Check sheet for the modelled part. Datum: model origin and axes. Units: mm. Face numbers are marked on the shaded views. A direction names the side the tool comes from. Give positions to 0.01 mm unless a question says otherwise; leave off trailing zeros. Loops run counter-clockwise (first coordinate to the right, second up) from the corner with the lowest first, then second, coordinate; pieces in that order, holes last. Notation, with made-up numbers: (-1.5, 11) -> (12.5, 11) arc R30 cw to (12.5, 47) -> close; hole circle Ø7 at (-5.75, 59.5). An arc over 180 degrees is marked (long way). Write each question's results on one line, items separated by ' | '. Start each with the question number.
Item 1: Scan lines: line 1 along Y through (x, z) = (23.5, 33); line 2 along Y through (x, z) = (1, 16); line 3 along Z through (x, y) = (-7, -13). Record each from-to range of solid material in increasing order.
Item 2: Cross-section at B-B on z = -7.5. Enter the section's corners in (x, y).
Item 3: Cross-section at C-C on x = 12.5. Enter the section's corners in (y, z).
Item 4: Access from +Z, -Z, +X, -X, +Y, -Y to the whole of each face (thin tool, end or side, straight path). Record for the marked faces 5, 6 and 7.
Item 5: Gauge pin test, flat ends, axial feed: pin 1 Ø6 at (y, z) = (-11.14, -7.5) entering from +X; pin 2 Ø0.9 at (x, y) = (33.5, -23) entering from +Z; pin 3 Ø7.5 at (x, z) = (30.5, -9) entering from +Y; pin 4 Ø3 at (x, z) = (33.81, -7.5) entering from -Y. Record the tip position at first contact, or that the pin passes through.
Item 6: Cross-section at D-D on z = 5.5. Enter the section's corners in (x, y), then the cut area to 3 significant figures.
Item 7: Cross-section at A-A on z = 39.5. Enter the section's corners in (x, y).
Item 8: Mould release check, pull along Y, two halves, no side actions. Record for the marked faces 1, 2, 3 and 4: pulls with the +Y half, pulls with the -Y half, needs draft (parallel to the pull), parting line crosses it, or undercut.
from build123d import *

# Parameters (mm, degrees)
SKETCH_1_W          = 42
SKETCH_1_H          = 61.5
EXTRUDE_1_DEPTH     = 3
SKETCH_2_W          = 42
SKETCH_2_H          = 9.2
SKETCH_2_H_2        = 2
EXTRUDE_2_DEPTH     = 42
SKETCH_3_R          = 12
SKETCH_3_R_2        = 1.65
CUT_EXTRUDE_1_DEPTH = 3
EXTRUDE_3_DEPTH     = 15
SKETCH_6_R          = 2.65
CUT_EXTRUDE_2_DEPTH = 5
SKETCH_7_W          = 15
SKETCH_7_H          = 3
EXTRUDE_4_DEPTH     = 20
SKETCH_8_R          = 2.65
CUT_EXTRUDE_3_DEPTH = 20


with BuildPart() as part:
    # 草图1 → 凸台-拉伸1 (new body)
    with BuildSketch(Plane.XY):
        with Locations((2.806034483, -19.390086207)):
            Rectangle(SKETCH_1_W, SKETCH_1_H)
    extrude(amount=EXTRUDE_1_DEPTH)

    # 草图2 → 凸台-拉伸2 (add)
    with BuildSketch(Plane.XY.offset(3)):
        with Locations((2.806034483, -45.540086207)):
            Rectangle(SKETCH_2_W, SKETCH_2_H)
        with Locations((2.806034483, 10.359913793)):
            Rectangle(SKETCH_2_W, SKETCH_2_H_2)
    extrude(amount=EXTRUDE_2_DEPTH)

    # 草图3 → 切除-拉伸1 (cut, through all)
    with BuildSketch(Plane.XZ.offset(-9.359913793)):
        with Locations((2.806034483, 24)):
            Circle(SKETCH_3_R)
        with Locations((18.306034483, 39.5)):
            Circle(SKETCH_3_R_2)
        with Locations((18.306034483, 8.5)):
            Circle(SKETCH_3_R_2)
        with Locations((-12.693965517, 8.5)):
            Circle(SKETCH_3_R_2)
        with Locations((-12.693965517, 39.5)):
            Circle(SKETCH_3_R_2)
    extrude(amount=-CUT_EXTRUDE_1_DEPTH, mode=Mode.SUBTRACT)

    # 草图4 → 凸台-拉伸3 (add)
    with BuildSketch(Plane(origin=(0, 0, 0), x_dir=(-1, 0, 0), z_dir=(0, 0, -1))):
        Polygon((-23.806034483, -21.140086207), (-23.806034483, -1.140086207), (-20.806034483, -1.140086207), (-20.806034483, -21.140086207), (-20.806034483, -24.140086207), (-23.806034483, -24.140086207), align=None)
    extrude(amount=EXTRUDE_3_DEPTH)

    # 草图6 → 切除-拉伸2 (cut)
    with BuildSketch(Plane.ZY.offset(-20.806034483)):
        with Locations((-7.5, -11.140086207)):
            Circle(SKETCH_6_R)
    extrude(amount=-CUT_EXTRUDE_2_DEPTH, mode=Mode.SUBTRACT)

    # 草图7 → 凸台-拉伸4 (add)
    with BuildSketch(Plane(origin=(23.806034483, 0, 0), x_dir=(0, 0, -1), z_dir=(1, 0, 0))):
        with Locations((7.5, -22.640086207)):
            Rectangle(SKETCH_7_W, SKETCH_7_H)
    extrude(amount=EXTRUDE_4_DEPTH)

    # 草图8 → 切除-拉伸3 (cut)
    with BuildSketch(Plane(origin=(0, -21.140086207, 0), x_dir=(1, 0, 0), z_dir=(0, 1, 0))):
        with Locations((33.806034483, 7.5)):
            Circle(SKETCH_8_R)
    extrude(amount=-CUT_EXTRUDE_3_DEPTH, mode=Mode.SUBTRACT)


solid = part.part
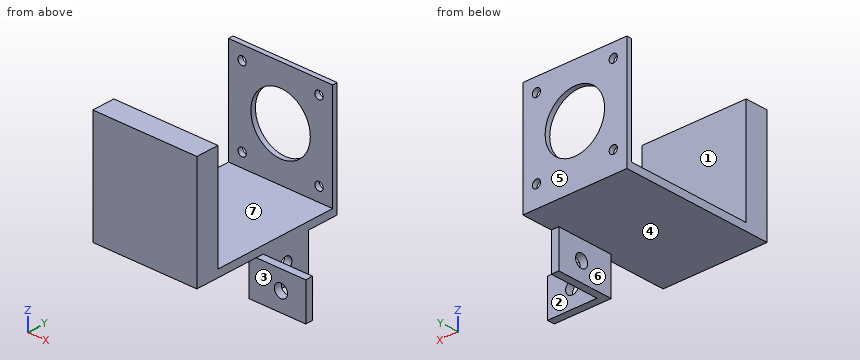
Answer sheet:
1) line 1: y = -50.14 to -40.94, 9.36 to 11.36 | line 2: y = -50.14 to -40.94 | line 3: z = 0 to 3
2) outline: (20.81, -24.14) -> (31.16, -24.14) -> (31.16, -21.14) -> (23.81, -21.14) -> (23.81, -13.79) -> (20.81, -13.79) -> close; (20.81, -8.49) -> (23.81, -8.49) -> (23.81, -1.14) -> (20.81, -1.14) -> close; (36.46, -24.14) -> (43.81, -24.14) -> (43.81, -21.14) -> (36.46, -21.14) -> close
3) outline: (-50.14, 0) -> (11.36, 0) -> (11.36, 16.93) -> (9.36, 16.93) -> (9.36, 3) -> (-40.94, 3) -> (-40.94, 45) -> (-50.14, 45) -> close; (9.36, 31.07) -> (11.36, 31.07) -> (11.36, 45) -> (9.36, 45) -> close
4) face 5: +Z, -Z, +X, -X, +Y | face 6: -Z, -X, +Y, -Y | face 7: +Z, +X, -X
5) pin 1: stops at x = 23.81 | pin 2: stops at z = 0 | pin 3: stops at y = -21.14 | pin 4: passes through
6) outline: (-18.19, -50.14) -> (23.81, -50.14) -> (23.81, -40.94) -> (-18.19, -40.94) -> close; (-18.19, 9.36) -> (23.81, 9.36) -> (23.81, 11.36) -> (-18.19, 11.36) -> close | area: 470 mm²
7) outline: (-18.19, -50.14) -> (23.81, -50.14) -> (23.81, -40.94) -> (-18.19, -40.94) -> close; (-18.19, 9.36) -> (-14.34, 9.36) -> (-14.34, 11.36) -> (-18.19, 11.36) -> close; (-11.04, 9.36) -> (16.66, 9.36) -> (16.66, 11.36) -> (-11.04, 11.36) -> close; (19.96, 9.36) -> (23.81, 9.36) -> (23.81, 11.36) -> (19.96, 11.36) -> close
8) face 1: undercut | face 2: pulls with the +Y half | face 3: pulls with the -Y half | face 4: needs draft
